```python
from build123d import *

# Parameters (mm, degrees)
SKETCH1_R                                            = 1.375
BOSS_EXTRUDE1_DEPTH                                  = 3
SKETCH2_R                                            = 3.5
SKETCH2_R_2                                          = 1.375
SKETCH2_R_3                                          = 4
BOSS_EXTRUDE2_DEPTH                                  = 5
SKETCH2_3_R                                          = 3.5
SKETCH2_3_R_2                                        = 1.375
BOSS_EXTRUDE3_DEPTH                                  = 5.3
SKETCH3_R                                            = 2.1
CUT_EXTRUDE1_DEPTH                                   = 102.373468088
CSK_FOR_M3_HEX_SOCKET_COUNTERSUNK_CAP_SC_D           = 3.6
CSK_FOR_M3_HEX_SOCKET_COUNTERSUNK_CAP_SC_DEPTH       = 14.44
CSK_FOR_M3_HEX_SOCKET_COUNTERSUNK_CAP_SC_CSINK_D     = 6.72
CSK_FOR_M3_HEX_SOCKET_COUNTERSUNK_CAP_SC_CSINK_ANGLE = 90
CSK_FOR_M3_HEX_SOCKET_COUNTERSUNK_CAP_SC_TIP         = 1.081549114
SKETCH6_W                                            = 40.311227037
SKETCH6_H                                            = 68
CUT_EXTRUDE2_DEPTH                                   = 102.172031867
FILLET1_R                                            = 6


with BuildPart() as part:
    # Sketch1 → Boss-Extrude1 (new body)
    # profile 1 of 3: a face of its own
    with BuildSketch(Plane.XY):
        with BuildLine():
            Line((-64.5, 35.5), (-64.5, 12.5))
            ThreePointArc((-64.5, 12.5), (-66.257359313, 8.257359313), (-70.5, 6.5))
            Line((-70.5, 6.5), (-78.424167346, 6.5))
            ThreePointArc((-78.424167346, 6.5), (-82.666808033, 4.742640687), (-84.424167346, 0.5))
            Line((-84.424167346, 0.5), (-84.424167346, -49.5))
            ThreePointArc((-84.424167346, -49.5), (-82.666808033, -53.742640687), (-78.424167346, -55.5))
            Line((-78.424167346, -55.5), (0.5, -55.5))
            ThreePointArc((0.5, -55.5), (4.742640687, -53.742640687), (6.5, -49.5))
            Line((6.5, -49.5), (6.5, 0.5))
            Line((6.5, 0.5), (6.5, 11.5))
            Line((6.5, 11.5), (6.5, 35.5))
            ThreePointArc((6.5, 35.5), (4.742640687, 39.742640687), (0.5, 41.5))
            Line((0.5, 41.5), (-58.5, 41.5))
            ThreePointArc((-58.5, 41.5), (-62.742640687, 39.742640687), (-64.5, 35.5))
        make_face()
        with BuildLine():
            ThreePointArc((0.5, -52.5), (2.621320344, -51.621320344), (3.5, -49.5))
            Line((3.5, -49.5), (3.5, 0.5))
            ThreePointArc((3.5, 0.5), (2.621320344, 2.621320344), (0.5, 3.5))
            Line((0.5, 3.5), (-78.424167346, 3.5))
            ThreePointArc((-78.424167346, 3.5), (-80.54548769, 2.621320344), (-81.424167346, 0.5))
            Line((-81.424167346, 0.5), (-81.424167346, -49.5))
            ThreePointArc((-81.424167346, -49.5), (-80.54548769, -51.621320344), (-78.424167346, -52.5))
            Line((-78.424167346, -52.5), (0.5, -52.5))
        make_face(mode=Mode.SUBTRACT)
        with BuildLine():
            ThreePointArc((-58.5, 38.5), (-60.621320344, 37.621320344), (-61.5, 35.5))
            Line((-61.5, 35.5), (-61.5, 11.5))
            ThreePointArc((-61.5, 11.5), (-60.621320344, 9.378679656), (-58.5, 8.5))
            Line((-58.5, 8.5), (0.5, 8.5))
            ThreePointArc((0.5, 8.5), (2.621320344, 9.378679656), (3.5, 11.5))
            Line((3.5, 11.5), (3.5, 35.5))
            ThreePointArc((3.5, 35.5), (2.621320344, 37.621320344), (0.5, 38.5))
            Line((0.5, 38.5), (-58.5, 38.5))
        make_face(mode=Mode.SUBTRACT)
    # profile 2 of 3: a face of its own
    with BuildSketch(Plane.XY):
        with BuildLine():
            Line((0.5, 38.5), (-58.5, 38.5))
            ThreePointArc((-58.5, 38.5), (-60.621320344, 37.621320344), (-61.5, 35.5))
            Line((-61.5, 35.5), (-61.5, 11.5))
            ThreePointArc((-61.5, 11.5), (-60.621320344, 9.378679656), (-58.5, 8.5))
            Line((-58.5, 8.5), (0.5, 8.5))
            ThreePointArc((0.5, 8.5), (2.621320344, 9.378679656), (3.5, 11.5))
            Line((3.5, 11.5), (3.5, 35.5))
            ThreePointArc((3.5, 35.5), (2.621320344, 37.621320344), (0.5, 38.5))
        make_face()
        with Locations((-58, 12)):
            Circle(SKETCH1_R, mode=Mode.SUBTRACT)
        with Locations((-58, 35)):
            Circle(SKETCH1_R, mode=Mode.SUBTRACT)
        with Locations((0, 35)):
            Circle(SKETCH1_R, mode=Mode.SUBTRACT)
        with Locations((0, 12)):
            Circle(SKETCH1_R, mode=Mode.SUBTRACT)
    # profile 3 of 3: a face of its own
    with BuildSketch(Plane.XY):
        with BuildLine():
            Line((-78.424167346, -52.5), (0.5, -52.5))
            ThreePointArc((0.5, -52.5), (2.621320344, -51.621320344), (3.5, -49.5))
            Line((3.5, -49.5), (3.5, 0.5))
            ThreePointArc((3.5, 0.5), (2.621320344, 2.621320344), (0.5, 3.5))
            Line((0.5, 3.5), (-78.424167346, 3.5))
            ThreePointArc((-78.424167346, 3.5), (-80.54548769, 2.621320344), (-81.424167346, 0.5))
            Line((-81.424167346, 0.5), (-81.424167346, -49.5))
            ThreePointArc((-81.424167346, -49.5), (-80.54548769, -51.621320344), (-78.424167346, -52.5))
        make_face()
        Circle(SKETCH1_R, mode=Mode.SUBTRACT)
        with Locations((0, -49)):
            Circle(SKETCH1_R, mode=Mode.SUBTRACT)
        with Locations((-58, -49)):
            Circle(SKETCH1_R, mode=Mode.SUBTRACT)
        with Locations((-58, 0)):
            Circle(SKETCH1_R, mode=Mode.SUBTRACT)
    extrude(amount=BOSS_EXTRUDE1_DEPTH)

    # Sketch2 → Boss-Extrude2 (add)
    # profile 1 of 4: a face of its own
    with BuildSketch(Plane.XY.offset(3)):
        with Locations((-58, 0)):
            Circle(SKETCH2_R)
        with Locations((-58, 0)):
            Circle(SKETCH2_R_2, mode=Mode.SUBTRACT)
    # profile 2 of 4: a face of its own
    with BuildSketch(Plane.XY.offset(3)):
        Circle(SKETCH2_R)
        Circle(SKETCH2_R_2, mode=Mode.SUBTRACT)
    # profile 3 of 4: a face of its own
    with BuildSketch(Plane.XY.offset(3)):
        with Locations((0, -49)):
            Circle(SKETCH2_R_3)
        with Locations((0, -49)):
            Circle(SKETCH2_R_2, mode=Mode.SUBTRACT)
    # profile 4 of 4: a face of its own
    with BuildSketch(Plane.XY.offset(3)):
        with Locations((-58, -49)):
            Circle(SKETCH2_R_3)
        with Locations((-58, -49)):
            Circle(SKETCH2_R_2, mode=Mode.SUBTRACT)
    extrude(amount=BOSS_EXTRUDE2_DEPTH)

    # Sketch2_3 → Boss-Extrude3 (add)
    # profile 1 of 4: a face of its own
    with BuildSketch(Plane.XY.offset(3)):
        with Locations((-58, 35)):
            Circle(SKETCH2_3_R)
        with Locations((-58, 35)):
            Circle(SKETCH2_3_R_2, mode=Mode.SUBTRACT)
    # profile 2 of 4: a face of its own
    with BuildSketch(Plane.XY.offset(3)):
        with Locations((-58, 12)):
            Circle(SKETCH2_3_R)
        with Locations((-58, 12)):
            Circle(SKETCH2_3_R_2, mode=Mode.SUBTRACT)
    # profile 3 of 4: a face of its own
    with BuildSketch(Plane.XY.offset(3)):
        with Locations((0, 35)):
            Circle(SKETCH2_3_R)
        with Locations((0, 35)):
            Circle(SKETCH2_3_R_2, mode=Mode.SUBTRACT)
    # profile 4 of 4: a face of its own
    with BuildSketch(Plane.XY.offset(3)):
        with Locations((0, 12)):
            Circle(SKETCH2_3_R)
        with Locations((0, 12)):
            Circle(SKETCH2_3_R_2, mode=Mode.SUBTRACT)
    extrude(amount=BOSS_EXTRUDE3_DEPTH)

    # Sketch3 → Cut-Extrude1 (cut, through all)
    with BuildSketch(Plane.XY.offset(8.3)):
        with Locations((-58, 35)):
            Circle(SKETCH3_R)
        with Locations((0, 35)):
            Circle(SKETCH3_R)
        with Locations((0, 12)):
            Circle(SKETCH3_R)
        with Locations((-58, 12)):
            Circle(SKETCH3_R)
        with Locations((-58, 0)):
            Circle(SKETCH3_R)
        Circle(SKETCH3_R)
        with Locations((-58, -49)):
            Circle(SKETCH3_R)
        with Locations((0, -49)):
            Circle(SKETCH3_R)
    extrude(amount=-CUT_EXTRUDE1_DEPTH, mode=Mode.SUBTRACT)

    # CSK for M3 Hex Socket Countersunk Cap Sc
    with Locations(Plane.XY.offset(3)):
        with Locations((-36.16376606, 6.225895505), (-21.164712778, 6.394420408)):
            CounterSinkHole(CSK_FOR_M3_HEX_SOCKET_COUNTERSUNK_CAP_SC_D / 2, CSK_FOR_M3_HEX_SOCKET_COUNTERSUNK_CAP_SC_CSINK_D / 2, depth=CSK_FOR_M3_HEX_SOCKET_COUNTERSUNK_CAP_SC_DEPTH, counter_sink_angle=CSK_FOR_M3_HEX_SOCKET_COUNTERSUNK_CAP_SC_CSINK_ANGLE)
            with Locations((0, 0, -(CSK_FOR_M3_HEX_SOCKET_COUNTERSUNK_CAP_SC_DEPTH + CSK_FOR_M3_HEX_SOCKET_COUNTERSUNK_CAP_SC_TIP / 2))):  # 118° drill point
                Cone(0, CSK_FOR_M3_HEX_SOCKET_COUNTERSUNK_CAP_SC_D / 2, CSK_FOR_M3_HEX_SOCKET_COUNTERSUNK_CAP_SC_TIP, mode=Mode.SUBTRACT)

    # Sketch6 → Cut-Extrude2 (cut, through all)
    with BuildSketch(Plane.XY.offset(3)):
        with Locations((-84.655613519, -21.5)):
            Rectangle(SKETCH6_W, SKETCH6_H)
    extrude(amount=-CUT_EXTRUDE2_DEPTH, mode=Mode.SUBTRACT)

    # Fillet1
    fillet1_edges = [part.edges().sort_by_distance(p)[0] for p in [
        (-64.5, -55.5, 1.5),
    ]]
    fillet(fillet1_edges, radius=FILLET1_R)


solid = part.part
```
Model file for the job. Use its own axes, mm. A direction names the side the tool comes from. Coordinates: 2 decimals unless noted, no trailing zeros. Write each loop counter-clockwise with the first axis right and the second up, starting at its lowest first coordinate (ties: lowest second). Pieces come first, ordered by that corner, then holes. Notation, with made-up numbers: (67.5, -9) - (99.5, -9) arc R26 ccw to (99.5, 16) - close; hole circle Ø6 at (14.25, 59). An arc over 180 degrees is marked (long way). One line per question, with ' | ' between items. Start each with the question number.
Q1. Drill centre lines: line 1 (Y direction, x = -58, z = 2.25); line 2 (Z direction, x = -53.5, y = 9); line 3 (X direction, y = 36, z = 1.5). Where is each one in solid material? Low to high. Write a range as [from, to].
Q2. Pin check, flat tips, straight feed: pin 1 (4 mm diameter, centred on x = -58, y = -49, fed in from +Z); pin 2 (2.5 mm diameter, centred on x = -0.5, y = -47.5, fed in from +Z); pin 3 (21.5 mm diameter, centred on x = -38, y = 11.5, fed in from +Z). Stop position of each tip, or through.
Q3. Pull direction X, two halves, no side cores. Call faces 1 (the face through (6.5, -8, 1)), 2 (the face through (-57.031, -50.863, 4.056)), 3 (the face through (-56, -51, 8)): pulls with the +X half, pulls with the -X half, needs draft (parallel to the pull), parting line crosses it, or undercut.
Q4. Cut at B-B, the plane x = -48.5. List the corners of the cut face in (y, z).
Q5. Cut at A-A, the plane z = 5. Give the number of separate pieces and of enclosed holes in the cut face, then the cut area to 3 significant figures.
Q6. Cut at C-C, the plane y = -25. List the corners of the cut face in (x, z).
Q7. 3-axis set-ups, long thin cutter, end or side, ignore diameter. For faces 4 (the face through (-54.185, -47.799, 5.465)), 5 (the face through (2, -51, 8)), 6 (the face through (-0.46, -51.05, 4.06)): which of +Z, -Z, +X, -X, +Y, -Y reach the whole face in a straight line?
Answer below:
1) line 1: [-55.5, -51.1], [-46.9, -2.1], [2.1, 9.9], [14.1, 32.9], [37.1, 41.5] | line 2: [0, 3] | line 3: [-64.48, -59.85], [-56.15, -1.85], [1.85, 6.48]
2) pin 1: through | pin 2: z = 8 | pin 3: z = 3
3) face 1: pulls with the +X half | face 2: undercut | face 3: needs draft
4) outline: (-55.5, 0) - (41.5, 0) - (41.5, 3) - (-55.5, 3) - close
5) separate pieces: 8 | enclosed holes: 8 | area: 221 mm^2
6) outline: (-64.5, 0) - (6.5, 0) - (6.5, 3) - (-64.5, 3) - close
7) face 4: +Z | face 5: +Z, +X, -X, -Y | face 6: +Z, -Z
